Autodesk Inventor part; units mm, degrees
ref_plane "YZ Plane" through (0, 0, 0) normal (1, 0, 0) x (0, 1, 0)
ref_plane "XZ Plane" through (0, 0, 0) normal (0, 1, 0) x (-1, 0, 0)
ref_plane "XY Plane" through (0, 0, 0) normal (0, 0, 1) x (1, 0, 0)
sketch "Boceto1" plane through (0, 0, 0) normal (0, 1, 0) x (-1, 0, 0)
  circle A0 centre (0, 0) radius 45
  circle A1 centre (0, 0) radius 54
  circle A2 centre (0, 0) radius 43
  dimension "d0" = 90
  dimension "d1" = 9
  dimension "d8" = 2
extrude "Extrusión1" add sketch "Boceto1" along normal blind 5 contours A0 | A1
sketch "Boceto2" plane through (0, 0, 0) normal (0, -1, 0) x (1, 0, 0)
  circle A0 centre (0, 0) radius 45
  circle A1 centre (0, 0) radius 43
  dimension "d7" = 2
extrude "Extrusión2" add sketch "Boceto2" along normal blind 38
sketch "Boceto3" plane through (0, -38, 0) normal (0, -1, 0) x (1, 0, 0)
  circle A0 centre (0, 0) radius 45
extrude "Extrusión3" add sketch "Boceto3" along normal blind 2
sketch "Boceto4" plane through (0, 5, 0) normal (0, 1, 0) x (1, 0, 0)
  circle A0 centre (0, 0) radius 45 construction
  circle A1 centre (0, 0) radius 49.5 construction
  circle A2 centre (-49.5, 0) radius 1.625
  circle A3 centre (0, 49.5) radius 1.625
  circle A4 centre (49.5, 0) radius 1.625
  circle A5 centre (0, -49.5) radius 1.625
  dimension "d11" = 4.5
  dimension "d12" = 90
  dimension "d13" = 3.25
  dimension "d14" = 3.25
  dimension "d15" = 3.25
  dimension "d16" = 3.25
extrude "Extrusión4" cut sketch "Boceto4" against normal blind 10
sketch "Boceto5" plane through (0, 5, 0) normal (0, 1, 0) x (1, 0, 0)
  circle A0 centre (0, 49.5) radius 1.625
  circle A1 centre (0, 49.5) radius 3
  circle A2 centre (49.5, 0) radius 1.625
  circle A3 centre (49.5, 0) radius 3
  circle A4 centre (0, -49.5) radius 1.625
  circle A5 centre (0, -49.5) radius 3
  circle A6 centre (-49.5, 0) radius 1.625
  circle A7 centre (-49.5, 0) radius 3
  point P0 (0, 0)
  dimension "d19" = 6
  dimension "d20" = 6
  dimension "d21" = 6
  dimension "d22" = 6
extrude "Extrusión5" cut sketch "Boceto5" against normal blind 2 contours A0 | A1 | A2 | A3 | A4 | A5 | A6 | A7
sketch "Boceto6" plane through (0, -40, 0) normal (0, -1, 0) x (1, 0, 0)
  circle A0 centre (0, 0) radius 13.125
  dimension "d33" = 26.25
extrude "Extrusión6" cut sketch "Boceto6" against normal blind 5
sketch "Boceto7" plane through (0, -38, 0) normal (0, 1, 0) x (1, 0, 0)
  circle A0 centre (0, 0) radius 13.125
  circle A1 centre (0, 0) radius 14.125
  dimension "d36" = 1
  dimension "d37" = 26.25
extrude "Extrusión7" add sketch "Boceto7" along normal blind 5
fillet "Empalme de cara1" radius 5 1 edges at (-14.125, -38, 0)
sketch "Boceto8" plane through (0, -40, 0) normal (0, -1, 0) x (1, 0, 0)
  line L0 (-102.7174, -0.1449) -> (97.2826, -0.1449)
  line L1 (97.2826, -0.1449) -> (97.2826, -10.1449)
  line L2 (97.2826, -10.1449) -> (-102.7174, -10.1449)
  line L3 (-102.7174, -10.1449) -> (-102.7174, -0.1449)
  point P0 (0, 0)
  dimension "d43" = 200
  dimension "d44" = 10
extrude "Extrusión8" add sketch "Boceto8" along normal blind 10
sketch "Boceto10" plane through (-102.7174, -40, -0.1449) normal (0, 0, 1) x (1, 0, 0)
  line L0 (57.7176, 0) -> (0, 0)
  line L1 (0, 0) -> (212.0347, 0)
  line L2 (156.7174, 45) -> (48.7174, 45)
  line L3 (48.7174, 45) -> (156.7174, 45)
  line L4 (102.7174, 45) -> (102.7174, 0) construction
  circle A0 centre (102.7174, 22.5) radius 9.55
  point P0 (102.7174, 40)
  dimension "d45" = 19.1
extrude "Extrusión9" cut sketch "Boceto10" along normal blind 70
sketch "Boceto11" plane through (0, -50, 0) normal (0, -1, 0) x (1, 0, 0)
  line L0 (-102.7174, -0.1449) -> (-102.7174, -10.1449)
  line L1 (-102.7174, -10.1449) -> (97.2826, -10.1449)
  line L2 (-102.7174, -0.1449) -> (97.2826, -0.1449)
  line L3 (97.2826, -0.1449) -> (97.2826, -10.1449)
  line L4 (97.2826, -10.1449) -> (-102.7174, -10.1449)
  line L5 (-102.7174, -10.1449) -> (-102.7174, -0.1449)
  point P0 (0, 0)
extrude "Extrusión10" cut sketch "Boceto11" against normal blind 10
Build history of the part. All positions in model axes, mm. A direction names the side the tool comes from. Round coordinates to 2 decimals unless told otherwise and drop trailing zeros. Order: outer loops, then holes, each group sorted by start corner. A loop starts at its lowest first (then second) coordinate and runs counter-clockwise, first axis right, second up. Notation, with made-up numbers: (47.5, 46) - (81.5, 46) arc R31 ccw to (81.5, 82) - close; hole circle Ø3 at (59, 59.25). An arc over 180 degrees is marked (long way). Use a Markdown table: item, result.
1) Tool access for faces 1 (the face through (9.1, -20.4, 43.4)), 2 (the face through (47.877, 1.521, -0.071)), 3 (the face through (-12, 0, -44)), 4 (the face through (9.4, -33, 9.4)): list every direction of +Z, -Z, +X, -X, +Y, -Y with a clear straight run to the whole face (end or side of a thin tool).
Recorded:
| item | result |
|---|---|
| face 1 | +Z |
| face 2 | +Y, -Y |
| face 3 | -Y |
| face 4 | +Y |
2) Pull direction X, two halves, no side cores. Call faces 5 (the face through (16.3, 5, 40.3)), 6 (the face through (-0.391, 4.014, 46.526)), 7 (the face through (20.765, -19.72, 39.923)): pulls with the +X half, pulls with the -X half, needs draft (parallel to the pull), parting line crosses it, or undercut.
Recorded:
| item | result |
|---|---|
| face 5 | needs draft |
| face 6 | undercut |
| face 7 | parting line crosses it |
3) Wall check: L1, parallel to Z at x = -6, y = -37; L2, parallel to Z at x = 0, y = -7; L3, parallel to Y at x = -18, z = -43. Give the ranges that are in metal, low to high.
Recorded:
| item | result |
|---|---|
| L1 | z = -44.6 to -42.58, -14.97 to -11.67, 11.67 to 14.97, 42.58 to 44.6 |
| L2 | z = -45 to -43, 43 to 45 |
| L3 | y = 0 to 5 |
4) Saw through at A-A on z = 49.5. Write the cut outline in (x, y) (3 decimals), and give its area (3 significant figures).
Recorded:
| item | result |
|---|---|
| outline | (-21.581, 0) - (-1.625, 0) - (-1.625, 3) - (-3, 3) - (-3, 5) - (-21.581, 5) - close; (1.625, 0) - (21.581, 0) - (21.581, 5) - (3, 5) - (3, 3) - (1.625, 3) - close |
| area | 194 mm² |
5) Saw through at C-C on x = -40. Write the cut outline in (y, z).
Recorded:
| item | result |
|---|---|
| outline | (-40, -20.62) - (0, -20.62) - (0, -36.28) - (5, -36.28) - (5, -15.78) - (-38, -15.78) - (-38, 15.78) - (5, 15.78) - (5, 36.28) - (0, 36.28) - (0, 20.62) - (-40, 20.62) - close |
6) Saw through at D-D on z = 0. Give the number of separate pieces and of enclosed holes in the cut face, and give its area (3 significant figures).
Recorded:
| item | result |
|---|---|
| separate pieces | 4 |
| enclosed holes | 0 |
| area | 367 mm² |
7) Flat gauge pins, fed straight in: pin 1 Ø11.5 at (x, y) = (0, -17.5) entering from +Z; pin 2 Ø4 at (x, z) = (16.5, -27.5) entering from +Y; pin 3 Ø4 at (x, z) = (0, 49.5) entering from -Y. Where does each tip first touch, or does it go through?
Recorded:
| item | result |
|---|---|
| pin 1 | stops at z = -42.61 |
| pin 2 | stops at y = -38 |
| pin 3 | stops at y = 0 |
8) Saw through at B-B on x = 49.5. Write the cut outline in (y, z) (3 decimals).
Recorded:
| item | result |
|---|---|
| outline | (0, -21.581) - (5, -21.581) - (5, -3) - (3, -3) - (3, -1.625) - (0, -1.625) - close; (0, 1.625) - (3, 1.625) - (3, 3) - (5, 3) - (5, 21.581) - (0, 21.581) - close |
